Read the model definition and answer for the solid it produces. Units are mm, in the model's axes. A direction names the side the tool comes from. Round coordinates to 2 decimals unless told otherwise and drop trailing zeros. Write each loop counter-clockwise with the first axis right and the second up, starting at its lowest first coordinate (ties: lowest second). Pieces come first, ordered by that corner, then holes. Notation, with made-up numbers: (21, 73) -> (67, 73) arc R23 cw to (67, 98) -> close; hole circle Ø7 at (26, 31). An arc over 180 degrees is marked (long way). Return JSON: item names as keys, results as strings. Group by question number.
(1) Straight lines are drawn through the part: line 1 (Z direction, x = 85, y = -0.85); line 2 (X direction, y = -0.95, z = -47.5); line 3 (Z direction, x = 14, y = -1.55). For each, find the intervals that lie inside material, in ascending order.
(2) A cutting plane is placed at C-C on y = -0.5. State how many separate pieces and enclosed holes the cut face has, then the cut area to 3 significant figures.
(3) For faces 1 (the flat face through (59, -2, -20)), 2 (the cylindrical face through (1.086, -1.565, -68.854)), determine the directions among +Z, -Z, +X, -X, +Y, -Y from which every point of the face is accessible in a straight line to the end or side of a thin tool.
(4) The mould has two halves that part along Z. Classify faces 3 (the cylindrical face through (118.854, -1.565, -68.914)), 4 (the flat face through (59, 0, -19)), 5 (the flat face through (61, -2, 0)), 6 (the cylindrical face through (34.792, -1.565, -63.414)): released by +Z, released by -Z, zero draft, split by the parting line, or undercut.
(5) A cutting plane is placed at A-A on x = 75. Give the vertices of the cut face in (y, z) (3 decimals).
(6) A cutting plane is placed at B-B on z = -29.5. Give the vertices of the cut face in (x, y) (3 decimals).
```python
from build123d import *

# Parameters (mm, degrees)
F0_R     = 1.6
F0_W     = 80
F0_H     = 30
F1_DEPTH = 3.175


with BuildPart() as f1:
    # F0 (on Front) → F1 (new body)
    with BuildSketch(Plane.XZ):
        with BuildLine():
            Line((116.19, 0), (3.81, 0))
            ThreePointArc((3.81, 0), (1.115923, -1.115923), (0, -3.81))
            Line((0, -3.81), (0, -66.19))
            ThreePointArc((0, -66.19), (1.115923, -68.884077), (3.81, -70))
            Line((3.81, -70), (116.19, -70))
            ThreePointArc((116.19, -70), (118.884077, -68.884077), (120, -66.19))
            Line((120, -66.19), (120, -3.81))
            ThreePointArc((120, -3.81), (118.884077, -1.115923), (116.19, 0))
        make_face()
        with Locations((5, -65)):
            Circle(F0_R, mode=Mode.SUBTRACT)
        with Locations((15, -65)):
            Circle(F0_R, mode=Mode.SUBTRACT)
        with Locations((25, -65)):
            Circle(F0_R, mode=Mode.SUBTRACT)
        with Locations((5, -55)):
            Circle(F0_R, mode=Mode.SUBTRACT)
        with Locations((16, -54.1)):
            Circle(F0_R, mode=Mode.SUBTRACT)
        with Locations((35, -65)):
            Circle(F0_R, mode=Mode.SUBTRACT)
        with Locations((45, -65)):
            Circle(F0_R, mode=Mode.SUBTRACT)
        with Locations((55, -65)):
            Circle(F0_R, mode=Mode.SUBTRACT)
        with Locations((5, -45)):
            Circle(F0_R, mode=Mode.SUBTRACT)
        with Locations((65, -65)):
            Circle(F0_R, mode=Mode.SUBTRACT)
        with Locations((75, -65)):
            Circle(F0_R, mode=Mode.SUBTRACT)
        with Locations((85, -65)):
            Circle(F0_R, mode=Mode.SUBTRACT)
        with Locations((95, -65)):
            Circle(F0_R, mode=Mode.SUBTRACT)
        with Locations((105, -65)):
            Circle(F0_R, mode=Mode.SUBTRACT)
        with Locations((115, -65)):
            Circle(F0_R, mode=Mode.SUBTRACT)
        with Locations((104, -54.1)):
            Circle(F0_R, mode=Mode.SUBTRACT)
        with Locations((115, -55)):
            Circle(F0_R, mode=Mode.SUBTRACT)
        with Locations((115, -45)):
            Circle(F0_R, mode=Mode.SUBTRACT)
        with Locations((5, -35)):
            Circle(F0_R, mode=Mode.SUBTRACT)
        with Locations((5, -25)):
            Circle(F0_R, mode=Mode.SUBTRACT)
        with Locations((5, -15)):
            Circle(F0_R, mode=Mode.SUBTRACT)
        with Locations((15.44, -15.9)):
            Circle(F0_R, mode=Mode.SUBTRACT)
        with Locations((5, -5)):
            Circle(F0_R, mode=Mode.SUBTRACT)
        with Locations((15, -5)):
            Circle(F0_R, mode=Mode.SUBTRACT)
        with Locations((25, -5)):
            Circle(F0_R, mode=Mode.SUBTRACT)
        with Locations((35, -5)):
            Circle(F0_R, mode=Mode.SUBTRACT)
        with Locations((45, -5)):
            Circle(F0_R, mode=Mode.SUBTRACT)
        with Locations((55, -5)):
            Circle(F0_R, mode=Mode.SUBTRACT)
        with Locations((60, -35)):
            Rectangle(F0_W, F0_H, mode=Mode.SUBTRACT)
        with Locations((115, -35)):
            Circle(F0_R, mode=Mode.SUBTRACT)
        with Locations((115, -25)):
            Circle(F0_R, mode=Mode.SUBTRACT)
        with Locations((65, -5)):
            Circle(F0_R, mode=Mode.SUBTRACT)
        with Locations((75, -5)):
            Circle(F0_R, mode=Mode.SUBTRACT)
        with Locations((85, -5)):
            Circle(F0_R, mode=Mode.SUBTRACT)
        with Locations((104, -15)):
            Circle(F0_R, mode=Mode.SUBTRACT)
        with Locations((115, -15)):
            Circle(F0_R, mode=Mode.SUBTRACT)
        with Locations((95, -5)):
            Circle(F0_R, mode=Mode.SUBTRACT)
        with Locations((105, -5)):
            Circle(F0_R, mode=Mode.SUBTRACT)
        with Locations((115, -5)):
            Circle(F0_R, mode=Mode.SUBTRACT)
    extrude(amount=F1_DEPTH)


solid = f1.part
```
Checks:
{
 "1": {"line 1": "z = -70 to -66.6, -63.4 to -50, -20 to -6.6, -3.4 to 0", "line 2": "x = 0 to 20, 100 to 120", "line 3": "z = -70 to -66.25, -63.75 to -16.6, -15.2 to -6.25, -3.75 to 0"},
 "2": {"separate pieces": "1", "enclosed holes": "39", "area": "5,680 mm^2"},
 "3": {"face 1": "+Y, -Y", "face 2": "-Z, -X, +Y, -Y"},
 "4": {"face 3": "released by -Z", "face 4": "zero draft", "face 5": "released by +Z", "face 6": "undercut"},
 "5": {"outline": "(-3.175, -70) -> (0, -70) -> (0, -66.6) -> (-3.175, -66.6) -> close; (-3.175, -63.4) -> (0, -63.4) -> (0, -50) -> (-3.175, -50) -> close; (-3.175, -20) -> (0, -20) -> (0, -6.6) -> (-3.175, -6.6) -> close; (-3.175, -3.4) -> (0, -3.4) -> (0, 0) -> (-3.175, 0) -> close"},
 "6": {"outline": "(0, -3.175) -> (20, -3.175) -> (20, 0) -> (0, 0) -> close; (100, -3.175) -> (120, -3.175) -> (120, 0) -> (100, 0) -> close"}
}
